Work out the finished part from the listing and answer in its coordinate system (mm). A direction names the side the tool comes from. Coordinates: 2 decimals unless noted, no trailing zeros. Loops run counter-clockwise (first coordinate to the right, second up) from the corner with the lowest first, then second, coordinate; pieces in that order, holes last. Notation, with made-up numbers: (-14.5, -12) -> (36.5, -12) arc R15 ccw to (36.5, 17) -> close; hole circle Ø8 at (51, 61). An arc over 180 degrees is marked (long way). One line per question, with ' | ' between items.
```python
from build123d import *

# Parameters (mm, degrees)
SKETCH_1_R                  = 2.75
EXTRUDE_1_DEPTH             = 35
SKETCH_2_R                  = 2.75
EXTRUDE_2_DEPTH             = 42
HOLE_WIZARD_3_5_3_5_1_D     = 3.5
HOLE_WIZARD_3_5_3_5_1_DEPTH = 13
HOLE_WIZARD_3_5_3_5_1_TIP   = 1.051506083
SKETCH_4_W                  = 0.8
SKETCH_4_H                  = 0.8
CUT_EXTRUDE_1_DEPTH         = 10
SKETCH_5_R                  = 3.5
EXTRUDE_3_DEPTH             = 6
CUT_EXTRUDE_2_DEPTH         = 1.5
SKETCH_7_R                  = 2
CUT_EXTRUDE_3_DEPTH         = 7
M2_5X0_451_D                = 2.05
M2_5X0_451_DEPTH            = 6
M2_5X0_451_TIP              = 0.615882135


with BuildPart() as part:
    # Эскиз1 → Бобышка-Вытянуть1 (new body)
    with BuildSketch(Plane(origin=(0, 0, 0), x_dir=(0, 0, -1), z_dir=(1, 0, 0))):
        Circle(SKETCH_1_R)
    extrude(amount=EXTRUDE_1_DEPTH)

    # Эскиз2 → Бобышка-Вытянуть2 (add)
    with BuildSketch(Plane(origin=(0, 0, 0), x_dir=(1, 0, 0), z_dir=(0, 1, 0))):
        with Locations((17.5, 0)):
            Circle(SKETCH_2_R)
    extrude(amount=EXTRUDE_2_DEPTH)

    # Диаметр отверстия Ø3.5 (3.5)1
    with Locations(Plane(origin=(17.5, 42, 0), x_dir=(0, 0, 1), z_dir=(0, 1, 0))):
        with Locations((0, 0)):
            Hole(HOLE_WIZARD_3_5_3_5_1_D / 2, depth=HOLE_WIZARD_3_5_3_5_1_DEPTH)
            with Locations((0, 0, -(HOLE_WIZARD_3_5_3_5_1_DEPTH + HOLE_WIZARD_3_5_3_5_1_TIP / 2))):  # 118° drill point
                Cone(0, HOLE_WIZARD_3_5_3_5_1_D / 2, HOLE_WIZARD_3_5_3_5_1_TIP, mode=Mode.SUBTRACT)

    # Эскиз4 → Вырез-Вытянуть1 (cut)
    with BuildSketch(Plane(origin=(0, 42, 0), x_dir=(1, 0, 0), z_dir=(0, 1, 0))):
        with BuildLine():
            Line((17.1, 4), (17.1, 2.720753572))
            ThreePointArc((17.1, 2.720753572), (17.5, 2.75), (17.9, 2.720753572))
            Line((17.9, 2.720753572), (17.9, 4))
            Line((17.9, 4), (17.1, 4))
        make_face()
        with BuildLine():
            Line((17.1, -1.703672504), (17.1, -2.720753572))
            ThreePointArc((17.1, -2.720753572), (17.5, -2.75), (17.9, -2.720753572))
            Line((17.9, -2.720753572), (17.9, -1.703672504))
            ThreePointArc((17.9, -1.703672504), (17.5, -1.75), (17.1, -1.703672504))
        make_face()
        with BuildLine():
            ThreePointArc((17.9, 2.720753572), (17.5, 2.75), (17.1, 2.720753572))
            Line((17.1, 2.720753572), (17.1, 1.703672504))
            ThreePointArc((17.1, 1.703672504), (17.5, 1.75), (17.9, 1.703672504))
            Line((17.9, 1.703672504), (17.9, 2.720753572))
        make_face()
        with BuildLine():
            Line((17.1, 1.703672504), (17.1, 0.4))
            Line((17.1, 0.4), (17.9, 0.4))
            Line((17.9, 0.4), (17.9, 1.703672504))
            ThreePointArc((17.9, 1.703672504), (17.5, 1.75), (17.1, 1.703672504))
        make_face()
        with Locations((17.5, 0)):
            Rectangle(SKETCH_4_W, SKETCH_4_H)
        with BuildLine():
            Line((15.796327496, -0.4), (17.1, -0.4))
            Line((17.1, -0.4), (17.1, 0.4))
            Line((17.1, 0.4), (15.796327496, 0.4))
            ThreePointArc((15.796327496, 0.4), (15.75, 0), (15.796327496, -0.4))
        make_face()
        with BuildLine():
            ThreePointArc((14.779246428, 0.4), (14.75, 0), (14.779246428, -0.4))
            Line((14.779246428, -0.4), (15.796327496, -0.4))
            ThreePointArc((15.796327496, -0.4), (15.75, 0), (15.796327496, 0.4))
            Line((15.796327496, 0.4), (14.779246428, 0.4))
        make_face()
        with BuildLine():
            Line((19.203672504, -0.4), (20.220753572, -0.4))
            ThreePointArc((20.220753572, -0.4), (20.242678647, -0.200533883), (20.25, 0))
            ThreePointArc((20.25, 0), (20.242678647, 0.200533883), (20.220753572, 0.4))
            Line((20.220753572, 0.4), (19.203672504, 0.4))
            ThreePointArc((19.203672504, 0.4), (19.238379545, 0.20133693), (19.25, 0))
            ThreePointArc((19.25, 0), (19.238379545, -0.20133693), (19.203672504, -0.4))
        make_face()
        with BuildLine():
            Line((13.5, -0.4), (14.779246428, -0.4))
            ThreePointArc((14.779246428, -0.4), (14.75, 0), (14.779246428, 0.4))
            Line((14.779246428, 0.4), (13.5, 0.4))
            Line((13.5, 0.4), (13.5, -0.4))
        make_face()
        with BuildLine():
            Line((17.1, -0.4), (17.1, -1.703672504))
            ThreePointArc((17.1, -1.703672504), (17.5, -1.75), (17.9, -1.703672504))
            Line((17.9, -1.703672504), (17.9, -0.4))
            Line((17.9, -0.4), (17.1, -0.4))
        make_face()
        with BuildLine():
            Line((17.1, -2.720753572), (17.1, -4))
            Line((17.1, -4), (17.9, -4))
            Line((17.9, -4), (17.9, -2.720753572))
            ThreePointArc((17.9, -2.720753572), (17.5, -2.75), (17.1, -2.720753572))
        make_face()
        with BuildLine():
            Line((17.9, 0.4), (17.9, -0.4))
            Line((17.9, -0.4), (19.203672504, -0.4))
            ThreePointArc((19.203672504, -0.4), (19.238379545, -0.20133693), (19.25, 0))
            ThreePointArc((19.25, 0), (19.238379545, 0.20133693), (19.203672504, 0.4))
            Line((19.203672504, 0.4), (17.9, 0.4))
        make_face()
        with BuildLine():
            ThreePointArc((20.25, 0), (20.242678647, -0.200533883), (20.220753572, -0.4))
            Line((20.220753572, -0.4), (21.5, -0.4))
            Line((21.5, -0.4), (21.5, 0.4))
            Line((21.5, 0.4), (20.220753572, 0.4))
            ThreePointArc((20.220753572, 0.4), (20.242678647, 0.200533883), (20.25, 0))
        make_face()
    extrude(amount=-CUT_EXTRUDE_1_DEPTH, mode=Mode.SUBTRACT)

    # Эскиз5 → Бобышка-Вытянуть3 (add)
    with BuildSketch(Plane(origin=(35, 0, 0), x_dir=(0, 0, -1), z_dir=(1, 0, 0))):
        Circle(SKETCH_5_R)
    extrude(amount=EXTRUDE_3_DEPTH)

    # Эскиз6 → Вырез-Вытянуть2 (cut)
    with BuildSketch(Plane(origin=(41, 0, 0), x_dir=(0, 0, -1), z_dir=(1, 0, 0))):
        with BuildLine():
            ThreePointArc((2.680951324, 2.25), (0, 3.5), (-2.680951324, 2.25))
            Line((-2.680951324, 2.25), (2.680951324, 2.25))
        make_face()
        with BuildLine():
            Line((2.680951324, -2.25), (-2.680951324, -2.25))
            ThreePointArc((-2.680951324, -2.25), (0, -3.5), (2.680951324, -2.25))
        make_face()
    extrude(amount=-CUT_EXTRUDE_2_DEPTH, mode=Mode.SUBTRACT)

    # Эскиз7 → Вырез-Вытянуть3 (cut)
    with BuildSketch(Plane.ZY):
        Circle(SKETCH_7_R)
    extrude(amount=-CUT_EXTRUDE_3_DEPTH, mode=Mode.SUBTRACT)

    # Отверстие обработанное метчиком M2.5x0.451
    with Locations(Plane(origin=(7, 0, 0), x_dir=(0, 0, -1), z_dir=(-1, 0, 0))):
        with Locations((0, 0)):
            Hole(M2_5X0_451_D / 2, depth=M2_5X0_451_DEPTH)
            with Locations((0, 0, -(M2_5X0_451_DEPTH + M2_5X0_451_TIP / 2))):  # 118° drill point
                Cone(0, M2_5X0_451_D / 2, M2_5X0_451_TIP, mode=Mode.SUBTRACT)


solid = part.part
```
1) For faces 1 (the face through (17.1, 37, -2)), 2 (the face through (39.5, 3, 0)), 3 (the face through (37.958, -3.105, -1.615)), determine the directions among +Z, -Z, +X, -X, +Y, -Y from which every point of the face is accessible in a straight line to the end or side of a thin tool.
Check values:
face 1: +Z, -Z, +Y | face 2: +Z, -Z, +X, +Y | face 3: +X
2) Find the intervals of material crossed by line 1 along Y through (x, z) = (4.5, 0); line 2 along Y through (x, z) = (8.9, 0) (3 decimals); line 3 along X through (y, z) = (38, 2), in increasing order.
Check values:
line 1: y = -2.75 to -2, 2 to 2.75 | line 2: y = -2.75 to -1.025, 1.025 to 2.75 | line 3: x = 15.61 to 17.1, 17.9 to 19.39
3) Find section A-A (y = 36). Write down the section's boundary in (x, z), plus the area to 3 significant figures.
Check values:
outline: (14.78, -0.4) arc R2.75 ccw to (17.1, -2.72) -> (17.1, -1.7) arc R1.75 cw to (15.8, -0.4) -> close; (14.78, 0.4) -> (15.8, 0.4) arc R1.75 cw to (17.1, 1.7) -> (17.1, 2.72) arc R2.75 ccw to start; (17.9, -2.72) arc R2.75 ccw to (20.22, -0.4) -> (19.2, -0.4) arc R1.75 cw to (17.9, -1.7) -> close; (17.9, 1.7) arc R1.75 cw to (19.2, 0.4) -> (20.22, 0.4) arc R2.75 ccw to (17.9, 2.72) -> close | area: 10.9 mm^2
4) Find section D-D (x = 3). Write down the section's boundary in (y, z).
Check values:
outline: circle Ø5.5 at (0, 0); hole circle Ø4 at (0, 0)
5) Flat-ended cylindrical pins translate along their axes: pin 1 (2 mm diameter, centred on y = 12.5, z = 1.5, fed in from +X); pin 2 (1 mm diameter, centred on y = 22.5, z = 1, fed in from -X); pin 3 (0.5 mm diameter, centred on y = 38.5, z = 2, fed in from -X). Find the tip coordinate at first contact, or state that the pin passes through.
Check values:
pin 1: stops at x = 20.2 | pin 2: stops at x = 14.8 | pin 3: stops at x = 15.38
6) Find section B-B (x = 8.5). Write down the section's boundary in (y, z) (3 decimals).
Check values:
outline: circle Ø5.5 at (0, 0); hole circle Ø2.05 at (0, 0)
7) The mould has two halves that part along Z. Classify faces 4 (the face through (20.04, 20.71, 1.05)), 5 (the face through (39.5, -3, 0)), 6 (the face through (10.042, -1.016, -0.133)): released by +Z, released by -Z, zero draft, split by the parting line, or undercut.
Check values:
face 4: split by the parting line | face 5: zero draft | face 6: undercut
8) Find section C-C (y = 25). Write down the section's boundary in (x, z).
Check values:
outline: circle Ø5.5 at (17.5, 0)
